The drawing under review shows one solid part. Ordinate dimensions are in mm from its lowest x, y, z. A direction names the side the tool comes from. Round coordinates to 2 decimals unless told otherwise and drop trailing zeros. Write each loop counter-clockwise with the first axis right and the second up, starting at its lowest first coordinate (ties: lowest second). Pieces come first, ordered by that corner, then holes. Notation, with made-up numbers: (-1.5, -20.75) -> (38.5, -20.75) arc R25 cw to (38.5, 6.25) -> close; hole circle Ø4 at (40, 61.5). An arc over 180 degrees is marked (long way). Use CSV: the item, a comma, the result in double quotes. Start each with the question number.
1) Take a section at D-D, the plane z = 33. Give the boundary of the cut face in (x, y) (1 decimal).
2) Take a section at A-A, the plane y = 8.5. Give the boundary of the cut face in (x, z) (1 decimal).
3) Wall thickness on probe 1 along Z at (x, y) = (2.05, 4.5) (1 decimal); probe 2 along X at (y, z) = (4.25, 41); probe 3 along X at (y, z) = (6.25, 21.5) (1 decimal): over which ranges is each line inside the solid? List them lowest first. Write a range as [from, to].
4) Take a section at B-B, the plane z = 19. Give the boundary of the cut face in (x, y), then the cut area to 3 significant figures.
5) Take a section at C-C, the plane x = 19. Give the boundary of the cut face in (y, z).
6) For pin 1 Ø1.5 at (x, y) = (12, 4.5) entering from -Z; pin 2 Ø5 at (x, y) = (9.5, 1.5) entering from +Z; pin 3 Ø5 at (x, y) = (6.5, 4.5) entering from +Z (1 decimal), all flat-tipped, find the tip position at first contact; note any pin that passes through.
7) Mouldability with a two-part tool opening along X and no side actions: class the marked faces 1, 2 and 3 as released by +X, released by -X, zero draft, split by the parting line, or undercut.
8) Machinability: for the marked faces 4 and 5, which of the approach directions +Z, -Z, +X, -X, +Y, -Y give a long, thin tool a straight path to every point of the face, cutting with its end or side? Answer none if there is none.
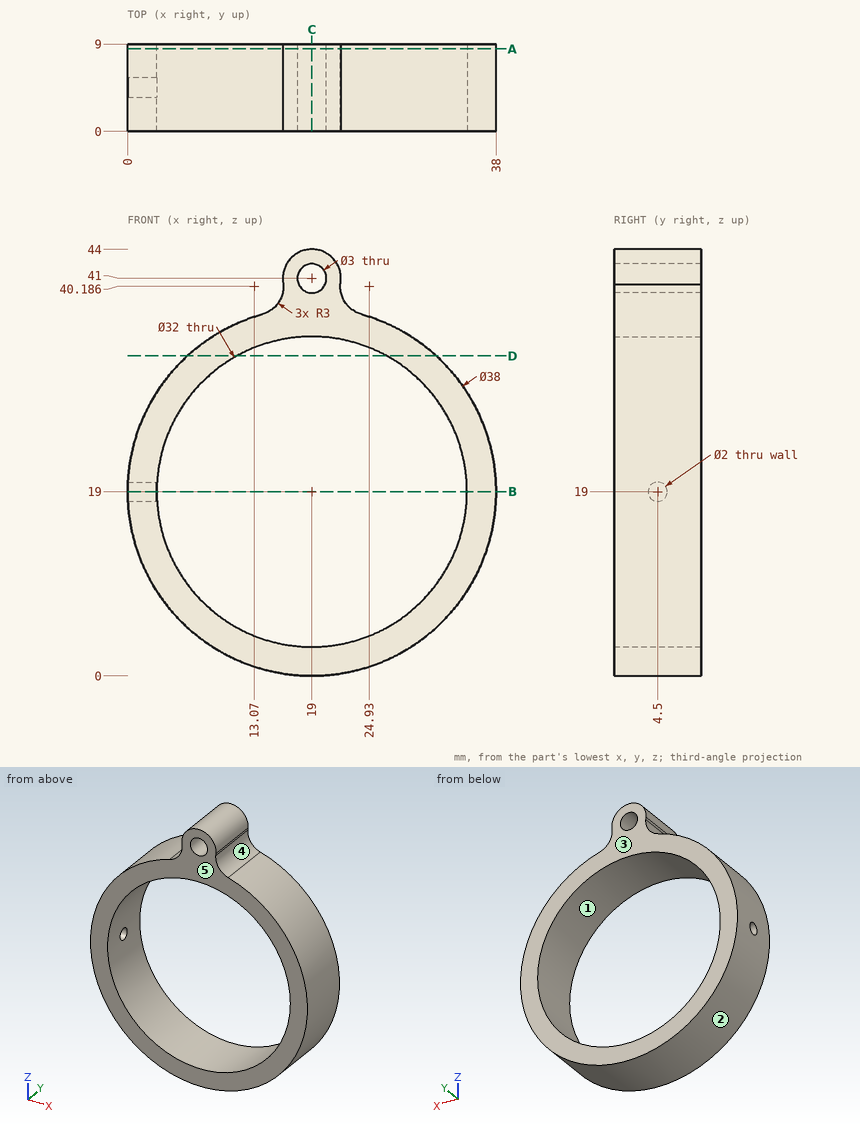
Values found:
1,outline,"(6.2, 0) -> (11.3, 0) -> (11.3, 9) -> (6.2, 9) -> close; (26.7, 0) -> (31.8, 0) -> (31.8, 9) -> (26.7, 9) -> close"
2,outline,"(13.9, 37.3) arc R19 ccw (long way) to (24.1, 37.3) arc R3 cw to (21.9, 40.4) arc R3 ccw (long way) to (16.1, 40.4) arc R3 cw to start; hole circle Ø32 at (19, 19); hole circle Ø3 at (19, 41)"
3,probe 1,"[10.4, 18], [20, 27.6]"
3,probe 2,"[16, 17.5], [20.5, 22]"
3,probe 3,"[0.2, 3.2], [34.8, 37.8]"
4,outline,"(0, 0) -> (3, 0) -> (3, 3.5) -> (0, 3.5) -> close; (0, 5.5) -> (3, 5.5) -> (3, 9) -> (0, 9) -> close; (35, 0) -> (38, 0) -> (38, 9) -> (35, 9) -> close"
4,area,"48.0 mm²"
5,outline,"(0, 0) -> (9, 0) -> (9, 3) -> (0, 3) -> close; (0, 35) -> (9, 35) -> (9, 39.5) -> (0, 39.5) -> close; (0, 42.5) -> (9, 42.5) -> (9, 44) -> (0, 44) -> close"
6,pin 1,"z = 1.06"
6,pin 2,"z = 36.66"
6,pin 3,"z = 35.2"
7,face 1,"undercut"
7,face 2,"split by the parting line"
7,face 3,"zero draft"
8,face 4,"+X, +Y, -Y"
8,face 5,"+Z, -Z, +X, -X, -Y"
